Check sheet for the modelled part. Datum: model origin and axes. Units: mm. Round coordinates to 2 decimals unless told otherwise and drop trailing zeros. Write each loop counter-clockwise with the first axis right and the second up, starting at its lowest first coordinate (ties: lowest second). Pieces come first, ordered by that corner, then holes. Notation, with made-up numbers: (-19.5, 86) -> (-10.5, 86) arc R15 ccw to (-10.5, 114) -> close; hole circle Ø4 at (89, 39). An arc over 180 degrees is marked (long way). One line per item, written item: value.
from build123d import *

# Parameters (mm, degrees)
F1_DEPTH = 40


with BuildPart() as f1:
    # F0 (on Top) → F1 (new body)
    with BuildSketch(Plane.XY):
        with BuildLine():
            ThreePointArc((7.3323928732, -1.5767101044), (5.4077667076, 0.2125573054), (7.1860144522, 2.1473696218))
            ThreePointArc((7.1860144522, 2.1473696218), (6.8110241928, 3.1400556437), (6.2996871297, 4.0698823162))
            ThreePointArc((6.2996871297, 4.0698823162), (3.673567798, 3.974169222), (3.5628599276, 6.5996991701))
            ThreePointArc((3.5628599276, 6.5996991701), (2.5957667546, 7.0364760325), (1.5767101044, 7.3323928732))
            ThreePointArc((1.5767101044, 7.3323928732), (-0.2125573054, 5.4077667076), (-2.1473696218, 7.1860144522))
            ThreePointArc((-2.1473696218, 7.1860144522), (-3.1400556437, 6.8110241928), (-4.0698823162, 6.2996871297))
            ThreePointArc((-4.0698823162, 6.2996871297), (-3.974169222, 3.673567798), (-6.5996991701, 3.5628599276))
            ThreePointArc((-6.5996991701, 3.5628599276), (-7.0364760325, 2.5957667546), (-7.3323928732, 1.5767101044))
            ThreePointArc((-7.3323928732, 1.5767101044), (-5.4077667076, -0.2125573054), (-7.1860144522, -2.1473696218))
            ThreePointArc((-7.1860144522, -2.1473696218), (-6.8110241928, -3.1400556437), (-6.2996871297, -4.0698823162))
            ThreePointArc((-6.2996871297, -4.0698823162), (-3.673567798, -3.974169222), (-3.5628599276, -6.5996991701))
            ThreePointArc((-3.5628599276, -6.5996991701), (-2.5957667546, -7.0364760325), (-1.5767101044, -7.3323928732))
            ThreePointArc((-1.5767101044, -7.3323928732), (0.2125573054, -5.4077667076), (2.1473696218, -7.1860144522))
            ThreePointArc((2.1473696218, -7.1860144522), (3.1400556437, -6.8110241928), (4.0698823162, -6.2996871297))
            ThreePointArc((4.0698823162, -6.2996871297), (3.974169222, -3.673567798), (6.5996991701, -3.5628599276))
            ThreePointArc((6.5996991701, -3.5628599276), (7.0364760325, -2.5957667546), (7.3323928732, -1.5767101044))
        make_face()
    extrude(amount=F1_DEPTH)


solid = f1.part
Item 1: Depth check by flat-ended pin: pin 1 (1.5 mm diameter, centred on x = -5, z = 31, fed in from -Y); pin 2 (8 mm diameter, centred on y = 4.5, z = 24, fed in from +X); pin 3 (3 mm diameter, centred on x = -5.5, z = 6.5, fed in from -Y). Enter the tip coordinate at first touch or a pass-through.
Result set:
pin 1: y = -3.67
pin 2: x = 7.19
pin 3: y = -4.07
Item 2: Sectioned sample at A-A (z = 24.5). Enter the section's corners in (x, y).
Result set:
outline: (-7.33, 1.58) arc R1.86 cw to (-7.19, -2.15) arc R7.5 ccw to (-6.3, -4.07) arc R1.86 cw to (-3.56, -6.6) arc R7.5 ccw to (-1.58, -7.33) arc R1.86 cw to (2.15, -7.19) arc R7.5 ccw to (4.07, -6.3) arc R1.86 cw to (6.6, -3.56) arc R7.5 ccw to (7.33, -1.58) arc R1.86 cw to (7.19, 2.15) arc R7.5 ccw to (6.3, 4.07) arc R1.86 cw to (3.56, 6.6) arc R7.5 ccw to (1.58, 7.33) arc R1.86 cw to (-2.15, 7.19) arc R7.5 ccw to (-4.07, 6.3) arc R1.86 cw to (-6.6, 3.56) arc R7.5 ccw to start
Item 3: Material ranges on line 1 along X through (y, z) = (6.25, 11.5); line 2 along X through (y, z) = (6.75, 10); line 3 along X through (y, z) = (0.25, 29) (3 decimals), recorded low to high.
Result set:
line 1: -4.02 to -1.85, 1.27 to 3.31
line 2: -3.27 to -2.08, 1.5 to 3.27
line 3: -5.485 to 5.407
Item 4: Sectioned sample at B-B (y = 0.75). Enter the section's corners in (x, z), then the cut area to 3 significant figures.
Result set:
outline: (-5.72, 0) -> (5.47, 0) -> (5.47, 40) -> (-5.72, 40) -> close
area: 447 mm^2
Item 5: Release check for a two-part mould opening along X. For faces 1 (the flat face through (0, 0, 40)), 2 (the cylindrical face through (3.127, -6.817, 19.72)), 3 (the cylindrical face through (3.95, -3.7, 19.72)) record: pulls with the +X half, pulls with the -X half, needs draft (parallel to the pull), parting line crosses it, or undercut.
Result set:
face 1: needs draft
face 2: pulls with the +X half
face 3: undercut
